Geometry: final body of the model. Coordinates: model frame, mm. A direction names the side the tool comes from. Give positions to 0.01 mm unless a question says otherwise; leave off trailing zeros. Order: outer loops, then holes, each group sorted by start corner. A loop starts at its lowest first (then second) coordinate and runs counter-clockwise, first axis right, second up. Notation, with made-up numbers: (29, 78.25) -> (41, 78.25) arc R27 ccw to (41, 104.25) -> close; hole circle Ø9 at (-9, 82). An arc over 180 degrees is marked (long way). Write item = value, one per line.
```python
from build123d import *

# Parameters (mm, degrees)
F0_W          = 63.5
F0_H          = 38.1
F1_DEPTH      = 6.35
F2_W          = 12.7
F2_H          = 29.21
F3_DEPTH      = 12.701
F5_DEPTH      = 6.35
F5_DEPTH_BACK = 6.35
F6_R          = 13.49375
F7_DEPTH      = 10.16
F8_R          = 11.43
F9_DEPTH      = 25.4
F11_D         = 7.1374


with BuildPart() as f1:
    # F0 (on Front) → F1 (new body, symmetric)
    with BuildSketch(Plane.XZ):
        Rectangle(F0_W, F0_H)
    extrude(amount=F1_DEPTH, both=True)

    # F2 (on face) → F3 (cut, through all)
    with BuildSketch(Plane.XZ.offset(6.35)):
        with Locations((-25.4, 4.445)):
            Rectangle(F2_W, F2_H)
        with Locations((25.4, 4.445)):
            Rectangle(F2_W, F2_H)
    extrude(amount=-F3_DEPTH, mode=Mode.SUBTRACT)

    # F4 (on Front) → F5 (join, two sides)
    with BuildSketch(Plane.XZ) as f5_sk:
        with BuildLine():
            Line((-19.05, 19.05), (19.05, 19.05))
            ThreePointArc((19.05, 19.05), (0, 38.1), (-19.05, 19.05))
        make_face()
    extrude(amount=F5_DEPTH)
    extrude(f5_sk.sketch, amount=-F5_DEPTH_BACK)

    # F6 (on face) → F7 (cut)
    with BuildSketch(Plane.XZ.offset(6.35)):
        with Locations((0, 19.05)):
            Circle(F6_R)
    extrude(amount=-F7_DEPTH, mode=Mode.SUBTRACT)

    # F8 (on face) → F9 (cut)
    with BuildSketch(Plane.XZ.offset(-3.81)):
        with Locations((0, 19.05)):
            Circle(F8_R)
    extrude(amount=-F9_DEPTH, mode=Mode.SUBTRACT)

    # F11 (through all)
    with Locations(Plane.XY.offset(-10.16)):
        with Locations((-25.4, 0), (25.4, 0)):
            Hole(F11_D / 2)


solid = f1.part
```
1) Line query: line 1 (Z direction, x = 0, y = 1.75); line 2 (Y direction, x = 25.4, z = -17); line 3 (X direction, y = 2, z = -5.5). Output: solid intervals per line, ascending. Write a range as from..to.
Check sheet entries:
line_1 = -19.05..5.56, 32.54..38.1
line_2 = -6.35..-3.57, 3.57..6.35
line_3 = -19.05..19.05
2) Section query C-C (z = 11). Output: boundary loops of the cut face in (x, y), plus the area to 3 significant figures.
Check sheet entries:
outline = (-19.05, -6.35) -> (-10.83, -6.35) -> (-10.83, 3.81) -> (-8.11, 3.81) -> (-8.11, 6.35) -> (-19.05, 6.35) -> close; (8.11, 3.81) -> (10.83, 3.81) -> (10.83, -6.35) -> (19.05, -6.35) -> (19.05, 6.35) -> (8.11, 6.35) -> close
area = 223 mm²
3) First-contact query: P1, Ø3, axis at x = 21, y = -2.5, coming from the +Z side; P2, Ø4, axis at y = -2.5, z = 2.5, coming from the +X side; P3, Ø1.5, axis at y = -4.5, z = 28.5, coming from the -X side; P4, Ø21.5, axis at x = 0, z = 19.05, coming from the -Y side. Flat tips, straight axial feed; report the tip coordinate or a pass-through.
Check sheet entries:
P1 = -10.16
P2 = 19.05
P3 = -16.95
P4 = through
4) Section query A-A (y = -2.25). Output: boundary loops of the cut face in (x, z).
Check sheet entries:
outline = (-31.75, -19.05) -> (-28.17, -19.05) -> (-28.17, -10.16) -> (-31.75, -10.16) -> close; (-22.63, -19.05) -> (22.63, -19.05) -> (22.63, -10.16) -> (19.05, -10.16) -> (19.05, 19.05) arc R19.05 ccw to (-19.05, 19.05) -> (-19.05, -10.16) -> (-22.63, -10.16) -> close; (28.17, -19.05) -> (31.75, -19.05) -> (31.75, -10.16) -> (28.17, -10.16) -> close; hole circle Ø26.99 at (0, 19.05)
5) Section query D-D (x = 25.4). Output: boundary loops of the cut face in (y, z), plus the area to 3 significant figures.
Check sheet entries:
outline = (-6.35, -19.05) -> (-3.57, -19.05) -> (-3.57, -10.16) -> (-6.35, -10.16) -> close; (3.57, -19.05) -> (6.35, -19.05) -> (6.35, -10.16) -> (3.57, -10.16) -> close
area = 49.5 mm²
6) Reachability of faces 5 (the face through (-28, 3, -10.16)), 6 (the face through (-2.93, -1.34, 5.88)), 7 (the face through (0.419, -0.089, 38.095)), 8 (the face through (0, 0, -19.05)), 9 (the face through (28, 3, -10.16)) from +Z, -Z, +X, -X, +Y, -Y: full face, straight path, thin tool, end or side. Return the list, or none.
Check sheet entries:
face_5 = +Z, -X, +Y, -Y
face_6 = -Y
face_7 = +Z, +Y, -Y
face_8 = -Z, +X, -X, +Y, -Y
face_9 = +Z, +X, +Y, -Y
7) Mould query, pull axis Y, two halves, no side actions, for faces 1 (the face through (-28.804, 1.072, -14.667)), 2 (the face through (0, -6.35, 4)), 3 (the face through (-31.75, 0, -15)), 4 (the face through (28.965, 0.157, -14.667)). Classes: +Y half, -Y half, draft (parallel to the pull), parting line (faces both ways), or undercut.
Check sheet entries:
face_1 = undercut
face_2 = -Y half
face_3 = draft
face_4 = undercut
8) Section query B-B (x = 0). Output: boundary loops of the cut face in (y, z), plus the area to 3 significant figures.
Check sheet entries:
outline = (-6.35, -19.05) -> (6.35, -19.05) -> (6.35, 7.62) -> (3.81, 7.62) -> (3.81, 5.56) -> (-6.35, 5.56) -> close; (-6.35, 32.54) -> (3.81, 32.54) -> (3.81, 30.48) -> (6.35, 30.48) -> (6.35, 38.1) -> (-6.35, 38.1) -> close
area = 394 mm²
